For this review, take the finished solid that the model builds, in its own axes (mm). Round coordinates to 2 decimals unless told otherwise and drop trailing zeros. Write each loop counter-clockwise with the first axis right and the second up, starting at its lowest first coordinate (ties: lowest second). Pieces come first, ordered by that corner, then holes. Notation, with made-up numbers: M -15.5,85 L 4.5,85 A4 cw 4.5,90 Z; hole C 6.5,-24 d9. An arc over 180 degrees is marked long. Write each question's results on one line, items separated by ' | '. Start each with the question number.
```python
from build123d import *

# Parameters (mm, degrees)
SKETCH1_W           = 508
SKETCH1_H           = 508
BOSS_EXTRUDE1_DEPTH = 25.4
FILLET1_R           = 12.7
FILLET2_R           = 12.7


with BuildPart() as part:
    # Sketch1 → Boss-Extrude1 (new body)
    with BuildSketch(Plane(origin=(0, 0, 0), x_dir=(1, 0, 0), z_dir=(0, 1, 0))):
        Rectangle(SKETCH1_W, SKETCH1_H)
    extrude(amount=BOSS_EXTRUDE1_DEPTH)

    # Fillet1
    fillet1_edges = [part.edges().sort_by_distance(p)[0] for p in [
        (-254, 25.4, 0),
        (0, 25.4, 254),
        (254, 25.4, 0),
        (0, 25.4, -254),
    ]]
    fillet(fillet1_edges, radius=FILLET1_R)

    # Fillet2
    # the kernel refuses this fillet: 12.7 mm, written as the material it takes off along each edge
    with BuildSketch(Plane(origin=(241.3, 12.7, 241.3), x_dir=(0, 0, 1), z_dir=(1, 0, 0))) as fillet2_piece_1_section:
        Polygon((0, 0), (FILLET2_R, 0), (FILLET2_R, -FILLET2_R), (0, -FILLET2_R), align=None)
    fillet2_piece_1 = extrude(amount=FILLET2_R, mode=Mode.PRIVATE)
    fillet2_piece_1 = fillet2_piece_1 - Plane(origin=(241.3, 12.7, 241.3), x_dir=(0, -0.7071067811865475, -0.7071067811865475), z_dir=(1, 0, 0)) * Sphere(FILLET2_R, mode=Mode.PRIVATE)
    add(fillet2_piece_1, mode=Mode.SUBTRACT)
    with BuildSketch(Plane(origin=(-241.3, 12.7, 241.3), x_dir=(0, 0, 1), z_dir=(-1, 0, 0))) as fillet2_piece_2_section:
        Polygon((0, 0), (FILLET2_R, 0), (FILLET2_R, FILLET2_R), (0, FILLET2_R), align=None)
    fillet2_piece_2 = extrude(amount=FILLET2_R, mode=Mode.PRIVATE)
    fillet2_piece_2 = fillet2_piece_2 - Plane(origin=(-241.3, 12.7, 241.3), x_dir=(0, -0.7071067811865475, -0.7071067811865475), z_dir=(-1, 0, 0)) * Sphere(FILLET2_R, mode=Mode.PRIVATE)
    add(fillet2_piece_2, mode=Mode.SUBTRACT)
    with BuildSketch(Plane(origin=(241.3, 12.7, -241.3), x_dir=(1, 0, 0), z_dir=(0, 0, -1))) as fillet2_piece_3_section:
        Polygon((0, 0), (FILLET2_R, 0), (FILLET2_R, -FILLET2_R), (0, -FILLET2_R), align=None)
    fillet2_piece_3 = extrude(amount=FILLET2_R, mode=Mode.PRIVATE)
    fillet2_piece_3 = fillet2_piece_3 - Plane(origin=(241.3, 12.7, -241.3), x_dir=(-0.7071067811865475, -0.7071067811865475, 0), z_dir=(0, 0, -1)) * Sphere(FILLET2_R, mode=Mode.PRIVATE)
    add(fillet2_piece_3, mode=Mode.SUBTRACT)
    with BuildSketch(Plane(origin=(-241.3, 12.7, -241.3), x_dir=(-1, 0, 0), z_dir=(0, 0, -1))) as fillet2_piece_4_section:
        Polygon((0, 0), (FILLET2_R, 0), (FILLET2_R, FILLET2_R), (0, FILLET2_R), align=None)
    fillet2_piece_4 = extrude(amount=FILLET2_R, mode=Mode.PRIVATE)
    fillet2_piece_4 = fillet2_piece_4 - Plane(origin=(-241.3, 12.7, -241.3), x_dir=(0.7071067811865475, -0.7071067811865475, 0), z_dir=(0, 0, -1)) * Sphere(FILLET2_R, mode=Mode.PRIVATE)
    add(fillet2_piece_4, mode=Mode.SUBTRACT)
    with BuildSketch(Plane(origin=(-254, -31.75, -254), x_dir=(1, 0, 0), z_dir=(0, 1, 0)), Plane(origin=(-254, -31.75, 254), x_dir=(0, 0, -1), z_dir=(0, 1, 0))) as fillet2_piece_5:
        with BuildLine():
            CenterArc((FILLET2_R, -FILLET2_R), FILLET2_R, 90, 90)
            Line((0, -FILLET2_R), (0, 0))
            Line((0, 0), (FILLET2_R, 0))
        make_face()
    extrude(amount=44.45, mode=Mode.SUBTRACT)
    with BuildSketch(Plane(origin=(254, -31.75, -254), x_dir=(-1, 0, 0), z_dir=(0, 1, 0)), Plane(origin=(254, -31.75, 254), x_dir=(0, 0, -1), z_dir=(0, 1, 0))) as fillet2_piece_6:
        with BuildLine():
            CenterArc((FILLET2_R, FILLET2_R), FILLET2_R, 180, 90)
            Line((0, FILLET2_R), (0, 0))
            Line((0, 0), (FILLET2_R, 0))
        make_face()
    extrude(amount=44.45, mode=Mode.SUBTRACT)


solid = part.part
```
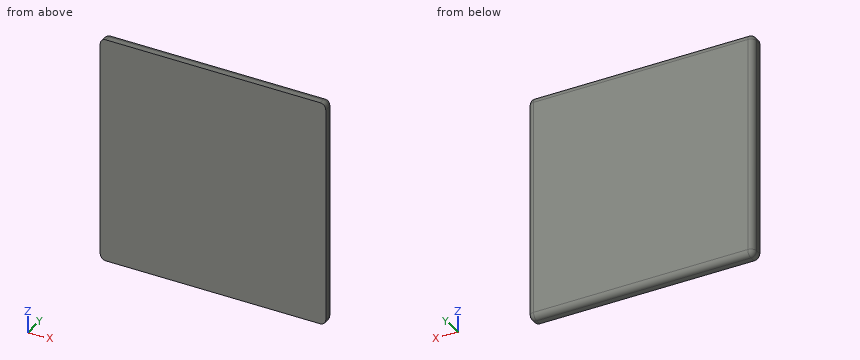
Item 1: For probe 1 along X at (y, z) = (14, -205); probe 2 along Z at (x, y) = (167, 16); probe 3 along Z at (x, y) = (-148, 16.25), list the stretches that pass through material, from the lowest coordinate up.
Item 2: We need section A-A on y = 19.5. State the section outline as (x, z) points, then the cut area to 3 significant figures.
Item 3: Insertion check: P1, Ø10, axis at y = 22.5, z = 47.5, coming from the +X side. The pin has a flat end and moves straight along its axis. Give the tip position at first contact, or say it passes through.
Numbers:
1) probe 1: x = -253.93 to 253.93 | probe 2: z = -253.56 to 253.56 | probe 3: z = -253.49 to 253.49
2) outline: M -252.03,-241.3 A10.73 ccw -241.3,-252.03 L 241.3,-252.03 A10.73 ccw 252.03,-241.3 L 252.03,241.3 A10.73 ccw 241.3,252.03 L -241.3,252.03 A10.73 ccw -252.03,241.3 Z | area: 254,000 mm^2
3) P1: stops at x = 253.06
